Answer from the drawing. Dimensions are ordinates in mm from the lowest x, y and z of the part. A direction names the side the tool comes from. Coordinates: 2 decimals unless noted, no trailing zeros. Write each loop counter-clockwise with the first axis right and the second up, starting at its lowest first coordinate (ties: lowest second). Pieces come first, ordered by that corner, then holes.
(1) The part is cut by section D-D, the plane z = 17.75. Determine the outline of the cut face in (x, y), and give its area (3 significant figures).
(2) The part is cut by section C-C, the plane x = 4.5. Determine the outline of the cut face in (y, z), and give its area (3 significant figures).
(3) Which of the six approach directions +Z, -Z, +X, -X, +Y, -Y give full straight-line access (tool end or side, diameter ignored) to the marked faces 1, 2 and 3?
(4) Determine the mould class of the marked faces 4, 5 and 6 for opening direction Y: pulls with the +Y half, pulls with the -Y half, needs draft (parallel to the pull), parting line crosses it, or undercut.
(5) Straight lines are drawn through the part: line 1 along Y through (x, z) = (20, 2.4); line 2 along Y through (x, z) = (1.5, 5.25). For each, find the intervals that lie inside material, in ascending order.
(6) The part is cut by section A-A, the plane x = 16. Determine the outline of the cut face in (y, z), and give its area (3 significant figures).
(7) The part is cut by section B-B, the plane z = 4. Determine the outline of the cut face in (x, y).
(8) Given pin 1 (3 mm diameter, centred on x = 11.5, y = 10.5, fed in from +Z); pin 2 (4 mm diameter, centred on x = 3, z = 17, fed in from +Y); pin 3 (4 mm diameter, centred on x = 7.5, z = 2.5, fed in from +Y); pin 4 (12 mm diameter, centred on x = 13, z = 5, fed in from -Y), each flat-ended and moving along its own axis, determine where each tip first touches the part or whether it passes through.
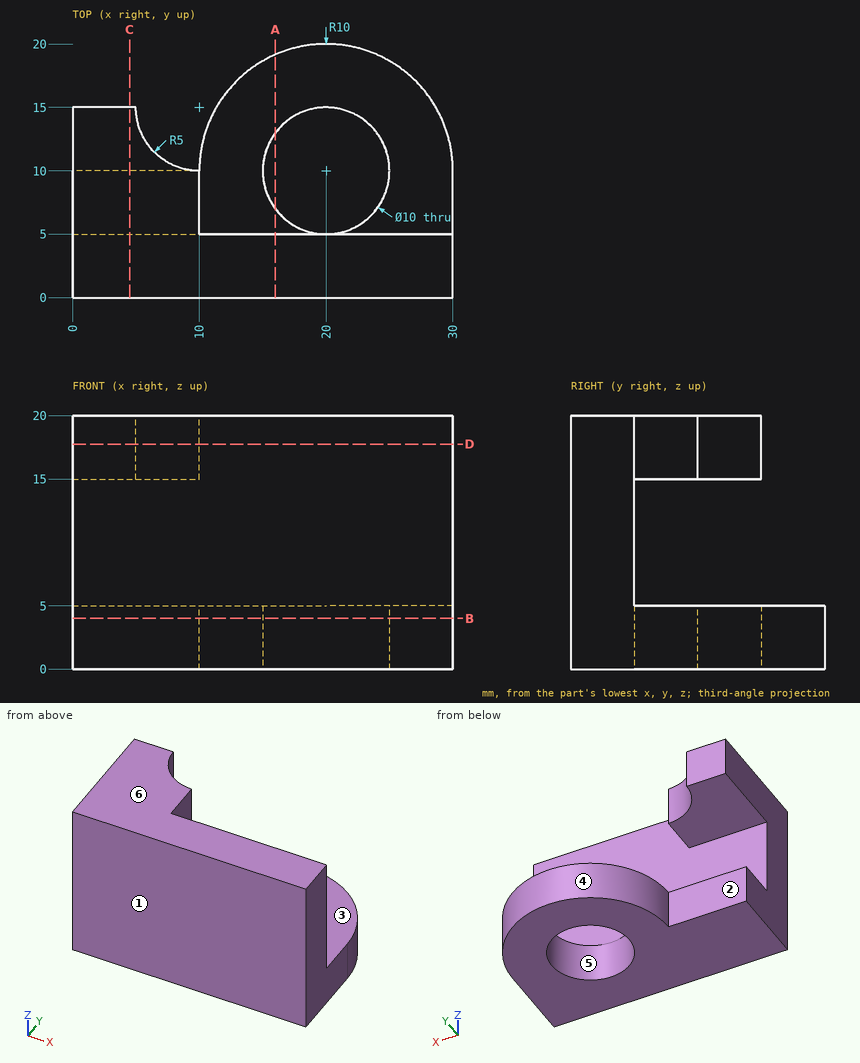
Computed:
1. outline: (0, 0) - (30, 0) - (30, 5) - (10, 5) - (10, 10) arc R5 cw to (5, 15) - (0, 15) - close
1. area: 230 mm2
2. outline: (0, 0) - (10, 0) - (10, 5) - (5, 5) - (5, 15) - (15, 15) - (15, 20) - (0, 20) - close
2. area: 175 mm2
3. face 1: +Z, -Z, +X, -X, -Y
3. face 2: -Z, -X, +Y
3. face 3: +X, -X, +Y
4. face 4: pulls with the +Y half
4. face 5: undercut
4. face 6: needs draft
5. line 1: y = 0 to 5, 15 to 20
5. line 2: y = 0 to 5
6. outline: (0, 0) - (7, 0) - (7, 5) - (5, 5) - (5, 20) - (0, 20) - close; (13, 0) - (19.17, 0) - (19.17, 5) - (13, 5) - close
6. area: 141 mm2
7. outline: (0, 0) - (30, 0) - (30, 10) arc R10 ccw to (10, 10) - (0, 10) - close; hole circle Ø10 at (20, 10)
8. pin 1: stops at z = 5
8. pin 2: stops at y = 15
8. pin 3: stops at y = 10
8. pin 4: stops at y = 0
